```python
from build123d import *

# Parameters (mm, degrees)
SKETCH4_W                = 47.7
SKETCH4_H                = 102.7
SKETCH4_W_2              = 35
SKETCH4_H_2              = 90
REVOLVE2_ANGLE           = 90
REVOLVE2_OTHER_WAY_ANGLE = 90
SKETCH10_W               = 102.7
SKETCH10_H               = 47.7
SKETCH10_W_2             = 90
SKETCH10_H_2             = 35
BOSS_EXTRUDE1_DEPTH      = 95
CUT_EXTRUDE2_DEPTH       = 360.751181374
SKETCH1_W                = 102.7
SKETCH1_H                = 47.7
SKETCH1_W_2              = 90
SKETCH1_H_2              = 35
CUT_EXTRUDE3_DEPTH       = 407.412084589
CUT_EXTRUDE3_DEPTH_BACK  = 407.412084589


with BuildPart() as part:
    # Sketch4 → Revolve2 (revolve)
    with BuildSketch(Plane(origin=(-16.35, 0, 0), x_dir=(0, -1, 0), z_dir=(-1, 0, 0))):
        with Locations((-141.5, -243.65)):
            Rectangle(SKETCH4_W, SKETCH4_H)
        with Locations((-141.5, -243.65)):
            Rectangle(SKETCH4_W_2, SKETCH4_H_2, mode=Mode.SUBTRACT)
    revolve(axis=Axis((-16.35, 289, -182.3), (0, -1, 0)), revolution_arc=REVOLVE2_ANGLE)

    # Sketch4 → Revolve2 other way (revolve)
    with BuildSketch(Plane(origin=(-16.35, 0, 0), x_dir=(0, -1, 0), z_dir=(-1, 0, 0))):
        with Locations((-141.5, -243.65)):
            Rectangle(SKETCH4_W, SKETCH4_H)
        with Locations((-141.5, -243.65)):
            Rectangle(SKETCH4_W_2, SKETCH4_H_2, mode=Mode.SUBTRACT)
    revolve(axis=Axis((-16.35, 289, -182.3), (0, 1, 0)), revolution_arc=REVOLVE2_OTHER_WAY_ANGLE)

    # Sketch10 → Boss-Extrude1 (add)
    with BuildSketch(Plane.XY.offset(-182.3)):
        with Locations((-77.7, 141.5)):
            Rectangle(SKETCH10_W, SKETCH10_H)
        with Locations((-77.7, 141.5)):
            Rectangle(SKETCH10_W_2, SKETCH10_H_2, mode=Mode.SUBTRACT)
    extrude(amount=BOSS_EXTRUDE1_DEPTH)

    # Sketch11 → Cut-Extrude2 (cut, through all)
    with BuildSketch(Plane(origin=(-26.35, 0, 0), x_dir=(0, 0, -1), z_dir=(1, 0, 0))):
        Polygon((87.3, 165.35), (87.3, 117.65), (129, 165.35), align=None)
    extrude(amount=-CUT_EXTRUDE2_DEPTH, mode=Mode.SUBTRACT)

    # Sweep1: sweep along a path in Sketch8
    with BuildLine(Plane(origin=(-6.35, 0, 0), x_dir=(0, -1, 0), z_dir=(-1, 0, 0))) as sweep1_path:
        ThreePointArc((5.835401436, 0), (-6.319346867, -52.292435279), (-40.291475749, -93.863232155))
        Line((-40.291475749, -93.863232155), (-94.90018434, -136.006572847))
        ThreePointArc((-94.90018434, -136.006572847), (-111.65526764, -156.509325764), (-117.65, -182.3))
    # Sketch1 → Sweep1 (sweep)
    with BuildSketch(Plane.XY):
        with Locations((45, 17.5)):
            Rectangle(SKETCH1_W, SKETCH1_H)
        with Locations((45, 17.5)):
            Rectangle(SKETCH1_W_2, SKETCH1_H_2, mode=Mode.SUBTRACT)
    sweep(path=sweep1_path.line)

    # Sketch12 → Cut-Extrude3 (cut, two sides: drawn at the far end of the back side and taken through both)
    with BuildSketch(Plane(origin=(96.35, 0, 0), x_dir=(0, 0, -1), z_dir=(1, 0, 0)).offset(-CUT_EXTRUDE3_DEPTH_BACK)):
        with BuildLine():
            Line((31.891429718, -2), (0, -2))
            Line((0, -2), (0, -6.35))
            ThreePointArc((0, -6.35), (16.093366564, -5.25748827), (31.891429718, -2))
        make_face()
        with BuildLine():
            Line((73.302994761, -2), (31.891429718, -2))
            ThreePointArc((31.891429718, -2), (16.093366564, -5.25748827), (0, -6.35))
            Line((0, -6.35), (73.302994761, -6.35))
            Line((73.302994761, -6.35), (73.302994761, -2))
        make_face()
    extrude(amount=CUT_EXTRUDE3_DEPTH + CUT_EXTRUDE3_DEPTH_BACK, mode=Mode.SUBTRACT)


solid = part.part
```
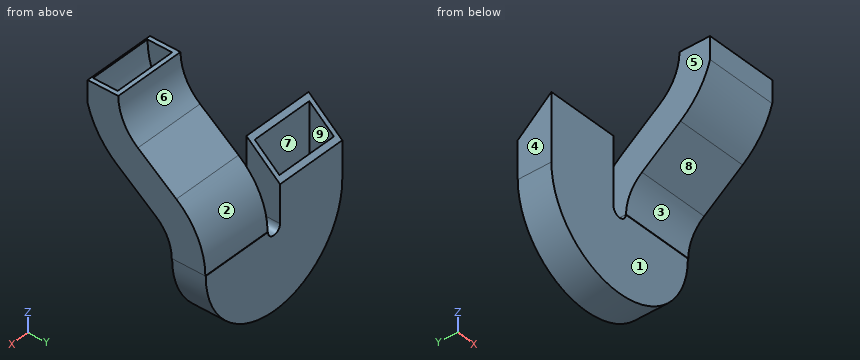
Can you work these out from the model? Positions are in its coordinate system, mm. Face numbers are marked on the shaded views. A direction names the side the tool comes from. Round coordinates to 2 decimals unless told otherwise and drop trailing zeros. Loops run counter-clockwise (first coordinate to the right, second up) from the corner with the lowest first, then second, coordinate; pieces in that order, holes last.
Item 1: Which directions (+Z, -Z, +X, -X, +Y, -Y) give clear straight access to the entire face, cutting with the end or side of a thin tool? Please do the marked faces 1, 2, 3, 4 and 5.
Item 2: Suppose I cut it at C-C, the plane y = 75. Write out the boundary of the cut face in (x, z), then the cut area to 3 significant figures.
Item 3: If we mould it in two halves opening along Z, with no side actions, what happens to the marked faces 6, 7, 8 and 9? For each: +Z half, -Z half, draft (parallel to the pull), parting line (faces both ways), or undercut.
Item 4: Suppose I cut it at B-B, the plane z = -107.5. Write out the boundary of the cut face in (x, y).
Item 5: Will these pins go through, and if not, where does the flat tip stop? pin 1 Ø0.6 at (x, y) = (43, 117.5) entering from -Z; pin 2 Ø3 at (x, z) = (-62, -167) entering from -Y; pin 3 Ø2 at (x, y) = (6.5, 48.5) entering from +Z.
Item 6: Please list where these lines run through material, in increasing order: L1, parallel to Y at x = -3, z = -208.5; L2, parallel to Y at x = -84, z = -97; L3, parallel to X at y = 6, z = -20.5.
Item 7: Suppose I cut it at D-D, the plane x = -102. Write out the boundary of the cut face in (y, z).
Item 8: Suppose I cut it at A-A, the plane x = -16.35. Write out the boundary of the cut face in (y, z), then the cut area to 3 significant figures.
Reported:
1. face 1: -Z, -X, -Y
1. face 2: +Z, +X, +Y
1. face 3: -Z, +X, -X, -Y
1. face 4: +Z, -Z, -X, +Y, -Y
1. face 5: +Z, +Y, -Y
2. outline: (-6.35, -121.3) - (96.35, -121.3) - (96.35, -61.05) - (-6.35, -61.05) - close; hole (0, -113.28) - (90, -113.28) - (90, -69.07) - (0, -69.07) - close
2. area: 2,210 mm2
3. face 6: +Z half
3. face 7: undercut
3. face 8: -Z half
3. face 9: draft
4. outline: (-129.05, 117.65) - (-26.35, 117.65) - (-26.35, 140.76) - (-32.7, 140.76) - (-32.7, 124) - (-122.7, 124) - (-122.7, 140.76) - (-129.05, 140.76) - close; (-6.35, 57.12) - (96.35, 57.12) - (96.35, 133.8) - (-6.35, 133.8) - close; hole (0, 67.51) - (90, 67.51) - (90, 124.5) - (0, 124.5) - close
5. pin 1: stops at z = -278.27
5. pin 2: stops at y = 117.65
5. pin 3: stops at z = -28.99
6. L1: y = 117.65 to 124, 159 to 165.35
6. L2: y = 117.65 to 124
6. L3: x = -6.35 to 0, 90 to 96.35
7. outline: (117.65, -255.55) - (165.35, -255.55) - (165.35, -129) - (159, -123.45) - (159, -245.34) - (124, -245.34) - (124, -92.85) - (117.65, -87.3) - close
8. outline: (117.65, -295) - (165.35, -295) - (165.35, -192.3) - (117.65, -192.3) - close; hole (124, -288.65) - (159, -288.65) - (159, -198.65) - (124, -198.65) - close
8. area: 1,750 mm2
